from build123d import *

# Parameters (mm, degrees)
CUT_EXTRUDE1_DEPTH      = 24.217586921
CUT_EXTRUDE1_DEPTH_BACK = 24.217586921
SKETCH4_R               = 2.032
FILLET1_R               = 0.09921875
CHAMFER1_SIZE           = 0.314729983


with BuildPart() as part:
    # Sketch3 → Revolve1 (revolve)
    with BuildSketch(Plane.XY, mode=Mode.PRIVATE) as revolve1_sk:
        with BuildLine():
            Line((-5.080939697, -3.02895), (-5.080939697, 4.437629646))
            Line((-5.080939697, 4.437629646), (-6.561510051, 5.9182))
            Line((-6.561510051, 5.9182), (-7.5057, 5.9182))
            Line((-7.5057, 5.9182), (-7.5057, -0.71755))
            ThreePointArc((-7.5057, -0.71755), (-8.351941732, -2.760558268), (-10.39495, -3.6068))
            Line((-10.39495, -3.6068), (-15.875, -3.6068))
            Line((-15.875, -3.6068), (-15.875, -5.9182))
            Line((-15.875, -5.9182), (-7.970189697, -5.9182))
            ThreePointArc((-7.970189697, -5.9182), (-5.927181429, -5.071958268), (-5.080939697, -3.02895))
        make_face()
    revolve(revolve1_sk.sketch.rotate(Axis((0, -5.9182, 0), (0, 1, 0)), 180), axis=Axis((0, -5.9182, 0), (0, 1, 0)))

    # Sketch4 → Cut-Extrude1 (cut, two sides: drawn at the far end of the back side and taken through both)
    with BuildSketch(Plane(origin=(0, 0, 0), x_dir=(1, 0, 0), z_dir=(0, 1, 0)).offset(-CUT_EXTRUDE1_DEPTH_BACK)):
        with Locations(Location((0, 12.303125, 0), (0, 0, 251.589901461))):
            Circle(SKETCH4_R)
        with Locations(Location((10.654818796, -6.1515625, 0), (0, 0, 131.589901463))):
            Circle(SKETCH4_R)
        with Locations(Location((-10.654818796, -6.1515625, 0), (0, 0, 48.410098537))):
            Circle(SKETCH4_R)
    extrude(amount=CUT_EXTRUDE1_DEPTH + CUT_EXTRUDE1_DEPTH_BACK, mode=Mode.SUBTRACT)

    # Fillet1
    fillet1_edges = [part.edges().sort_by_distance(p)[0] for p in [
        (-15.875, -5.9182, 0),
        (-15.875, -3.6068, 0),
    ]]
    fillet(fillet1_edges, radius=FILLET1_R)

    # Chamfer1
    chamfer1_edges = [part.edges().sort_by_distance(p)[0] for p in [
        (-7.5057, 5.9182, 0),
    ]]
    chamfer(chamfer1_edges, length=CHAMFER1_SIZE)


solid = part.part
For this review, take the finished solid that the model builds, in its own axes (mm). A direction names the side the tool comes from. Coordinates: 2 decimals unless noted, no trailing zeros. Order: outer loops, then holes, each group sorted by start corner. A loop starts at its lowest first (then second) coordinate and runs counter-clockwise, first axis right, second up. Notation, with made-up numbers: (-15, 43.25) - (33, 43.25) arc R26 cw to (33, 78.25) - close; hole circle Ø7 at (-27, 40). An arc over 180 degrees is marked (long way). Use one line per item in the form item = value.
Q1. For P1, Ø1.5, axis at x = -3.5, y = 1.5, coming from the +Z side; P2, Ø1.5, axis at x = 10, y = -4.5, coming from the +Z side; P3, Ø6.5, axis at x = 10.65, z = 6.15, coming from the +Y side, all flat-tipped, find the tip position at first contact; note any pin that passes through.
Checked values:
P1 = 6.98
P2 = 12.9
P3 = -3.27
Q2. Consider section B-B (x = 0). Give the number of separate pieces and of enclosed holes in the cut face, then the cut area to 3 significant figures.
Checked values:
separate_pieces = 3
enclosed_holes = 0
area = 84.4 mm2
Q3. Consider section D-D (y = 0.25). Give the boundary of the cut face in (x, z).
Checked values:
outline = circle Ø15.01 at (0, 0); hole circle Ø10.16 at (0, 0)
Q4. Consider section C-C (y = -4.25). Give the boundary of the cut face in (x, z) (3 decimals), then the cut area to 3 significant figures.
Checked values:
outline = circle Ø31.75 at (0, 0); hole circle Ø4.064 at (-10.655, 6.152); hole circle Ø10.703 at (0, 0); hole circle Ø4.064 at (0, -12.303); hole circle Ø4.064 at (10.655, 6.152)
area = 663 mm2
Q5. For probe 1 along Z at (x, y) = (-1.5, -4.5); probe 2 along Z at (x, y) = (0, -4.4) (3 decimals); probe 3 along Y at (x, z) = (-0.5, 11), list the stretches that pass through material, from the lowest coordinate up. Write a range as from..to.
Checked values:
probe_1 = -15.8..-13.67, -10.93..-5.27, 5.27..15.8
probe_2 = -15.875..-14.335, -10.271..-5.427, 5.427..15.875
probe_3 = -5.92..-3.61
Q6. Draft analysis for pull direction X (two halves, no side actions). For faces 1 (the flat face through (-6.4, 5.918, 2.1)), 2 (the cylindrical face through (12.65, -4.78, 6.54)), 3 (the cylindrical face through (-3.441, -4.777, 15.497)), state which applies: +X half, -X half, draft (parallel to the pull), parting line (faces both ways), or undercut.
Checked values:
face_1 = draft
face_2 = undercut
face_3 = parting line
Q7. For faces 4 (the cylindrical face through (-12.337, -4.777, 5.012)), 5 (the flat face through (-3.3, -3.607, 10.3)), list the 3-axis set-ups (+Z, -Z, +X, -X, +Y, -Y) from which the entire face can be reached by the end or side of a thin tool; tool diameter is ignored.
Checked values:
face_4 = +Y, -Y
face_5 = +Y
